Autodesk Inventor part; units mm, degrees
ref_plane "YZ Plane" through (0, 0, 0) normal (1, 0, 0) x (0, 1, 0)
ref_plane "XZ Plane" through (0, 0, 0) normal (0, 1, 0) x (-1, 0, 0)
ref_plane "XY Plane" through (0, 0, 0) normal (0, 0, 1) x (1, 0, 0)
sketch "Sketch1" plane through (0, 0, 0) normal (0, 0, 1) x (1, 0, 0)
  line L0 (-18.9528, 7.3952) -> (6.4472, 7.3952)
  line L1 (6.4472, 7.3952) -> (6.4472, -18.0048)
  line L2 (6.4472, -18.0048) -> (-18.9528, -18.0048)
  line L3 (-18.9528, -18.0048) -> (-18.9528, 7.3952)
  line L4 (-17.3653, 5.8077) -> (4.8597, 5.8077)
  line L5 (4.8597, 5.8077) -> (4.8597, -16.4173)
  line L6 (4.8597, -16.4173) -> (-17.3653, -16.4173)
  line L7 (-17.3653, -16.4173) -> (-17.3653, 5.8077)
  point P0 (0, 0)
  dimension "d0" = 25.4
  dimension "d1" = 25.4
  dimension "d2" = 1.5875
  dimension "d3" = 1.5875
  dimension "d4" = 1.5875
  dimension "d5" = 1.5875
extrude "Extrusion1" add sketch "Sketch1" along normal blind 50.8
properties part number "1-16 tube 2''"
Geometry check sheet. Reference: the model listing, model coordinates, mm. A direction names the side the tool comes from. Give positions to 0.01 mm unless a question says otherwise; leave off trailing zeros. Order: outer loops, then holes, each group sorted by start corner. A loop starts at its lowest first (then second) coordinate and runs counter-clockwise, first axis right, second up. Notation, with made-up numbers: (69.25, 11) - (126.25, 11) arc R12 ccw to (126.25, 26) - close; hole circle Ø8 at (11.5, 79). An arc over 180 degrees is marked (long way). Write item = value, one per line. Start each with the question number.
1) Section check B-B (z = 19.5). Enter the section's corners in (x, y).
2) Section check C-C (y = -7.5). Enter the section's corners in (x, z).
3) Section check A-A (x = 2.25). Enter the section's corners in (y, z).
4) Draft check along X on faces 1 (the flat face through (-17.365, -5, 25)), 2 (the flat face through (-18, -5, 50.8)), 3 (the flat face through (6.447, -5, 25)). Enter one of: released by +X, released by -X, zero draft, split by the parting line, or undercut.
5) Scan lines: L1, parallel to Y at x = -8.5, z = 36.5; L2, parallel to X at y = -2.5, z = 3. Record each from-to range of solid material in increasing order.
6) Access from +Z, -Z, +X, -X, +Y, -Y to the whole of each face (thin tool, end or side, straight path). Record for faces 4 (the flat face through (-6, 7.395, 25)), 5 (the flat face through (4.86, -5, 25)).
7) Gauge pin test, flat ends, axial feed: pin 1 Ø10 at (x, y) = (-4, -4.5) entering from -Z; pin 2 Ø12 at (x, y) = (0.5, -9.5) entering from -Z. Record the tip position at first contact, or that the pin passes through.
Geometry check:
q1.outline = (-18.95, -18) - (6.45, -18) - (6.45, 7.4) - (-18.95, 7.4) - close; hole (-17.37, -16.42) - (4.86, -16.42) - (4.86, 5.81) - (-17.37, 5.81) - close
q2.outline = (-18.95, 0) - (-17.37, 0) - (-17.37, 50.8) - (-18.95, 50.8) - close; (4.86, 0) - (6.45, 0) - (6.45, 50.8) - (4.86, 50.8) - close
q3.outline = (-18, 0) - (-16.42, 0) - (-16.42, 50.8) - (-18, 50.8) - close; (5.81, 0) - (7.4, 0) - (7.4, 50.8) - (5.81, 50.8) - close
q4.face_1 = undercut
q4.face_2 = zero draft
q4.face_3 = released by +X
q5.L1 = -18 to -16.42, 5.81 to 7.4
q5.L2 = -18.95 to -17.37, 4.86 to 6.45
q6.face_4 = +Z, -Z, +X, -X, +Y
q6.face_5 = +Z, -Z
q7.pin_1 = through
q7.pin_2 = 0
